```python
from build123d import *

# Parameters (mm, degrees)
BOSS_EXTRUDE1_DEPTH = 2


with BuildPart() as part:
    # Sketch1 → Boss-Extrude1 (new body)
    with BuildSketch(Plane(origin=(0, 0, 0), x_dir=(1, 0, 0), z_dir=(0, 1, 0))):
        with BuildLine():
            Line((-34.272006578, 2.022637666), (0.021174984, -25.087844423))
            Line((0.021174984, -25.087844423), (24.827751164, 6.291030289))
            Line((24.827751164, 6.291030289), (-9.465430397, 33.401512378))
            ThreePointArc((-9.465430397, 33.401512378), (-14.475065348, 35.485495243), (-19.835620944, 34.646525273))
            ThreePointArc((-19.835620944, 34.646525273), (-31.599371908, 25.404645185), (-37.876767257, 11.825525482))
            ThreePointArc((-37.876767257, 11.825525482), (-37.455913062, 6.416060752), (-34.272006578, 2.022637666))
        make_face()
    extrude(amount=BOSS_EXTRUDE1_DEPTH)


solid = part.part
```
Check sheet for the modelled part. Datum: model origin and axes. Units: mm. Round coordinates to 2 decimals unless told otherwise and drop trailing zeros. Order: outer loops, then holes, each group sorted by start corner. A loop starts at its lowest first (then second) coordinate and runs counter-clockwise, first axis right, second up.
1) Section check C-C (x = -23). Record the boundary of the cut face in (y, z).
2) Go/stop test with flat-tipped pins: pin 1 Ø10 at (x, z) = (-9, 0.5) entering from -Y; pin 2 Ø1 at (y, z) = (1.5, -13.5) entering from -X; pin 3 Ø1 at (x, y) = (16.5, 1.5) entering from -Z. Record where each tip stops, or that it passes through.
3) Section check A-A (y = 1.1). Record the boundary of the cut face in (x, z).
4) Scan lines: line 1 (X direction, y = 0.4, z = -11.5); line 2 (X direction, y = 0.2, z = -20.5); line 3 (Z direction, x = -19, y = 1.7). Record each from-to range of solid material in increasing order.
5) Section check B-B (z = 10). Record the boundary of the cut face in (x, y), and give its area (3 significant figures).
Result:
1. outline: (0, -32.98) - (2, -32.98) - (2, 6.89) - (0, 6.89) - close
2. pin 1: stops at y = 0
2. pin 2: stops at x = -37.62
2. pin 3: stops at z = -13.27
3. outline: (-37.88, -11.83) arc R32 ccw to (-19.84, -34.65) arc R10 ccw to (-9.47, -33.4) - (24.83, -6.29) - (0.02, 25.09) - (-34.27, -2.02) arc R10 ccw to start
4. line 1: x = -37.94 to 18.24
4. line 2: x = -34.79 to 6.85
4. line 3: z = -34.99 to 10.05
5. outline: (-19.06, 0) - (11.95, 0) - (11.95, 2) - (-19.06, 2) - close
5. area: 62.0 mm2
